Here's how the part is built. I have some questions about the finished solid (model axes, mm). A direction names the side the tool comes from. Give positions to 0.01 mm unless a question says otherwise; leave off trailing zeros. Loops run counter-clockwise (first coordinate to the right, second up) from the corner with the lowest first, then second, coordinate; pieces in that order, holes last.
Q1. If we section it at C-C (y = 32): Please give me the cut outline in (x, z) (3 decimals).
Q2. If we section it at D-D (z = -35.5): Please give me the cut outline in (x, y), plus the area to 3 significant figures.
Q3. If we section it at A-A (x = -12.5): Please give me the cut outline in (y, z) (3 decimals).
Q4. I need wall thicknesses on line 1 (X direction, y = 15, z = -4); line 2 (X direction, y = 8, z = -10); line 3 (Y direction, x = -12.5, z = -7.9). Which ranges of each line are inside material? Lowest first, please.
Q5. For faces 1 (the face through (-5, 13, -7.1)), 2 (the face through (-48, 28, -162)), 3 (the face through (-47, 28, -3)), 4 (the face through (-30, 32, -8)), which set-ups out of +Z, -Z, +X, -X, +Y, -Y let a thin tool reach every point of the face, with its end or its side?
Q6. We'd pull the mould along Y, two halves only. Please class faces 5 (the face through (-50, 33.75, -8)), 6 (the face through (-2, 13, -84)), 7 (the face through (-30, 32, -157)), 8 (the face through (-35, 30, -165)): +Y half, -Y half, draft (parallel to the pull), parting line (faces both ways), or undercut.
Q7. If we section it at B-B (y = 15.5): Give the number of separate pieces and of enclosed holes in the cut face, plus the area to 3 significant figures.
Q8. Will these pins go through, and if not, where does the flat tip stop? P1, Ø1, axis at x = -18.5, y = 7.5, coming from the -Z side; P2, Ø2.5, axis at x = -1, z = -106, coming from the +Y side; P3, Ø12, axis at y = 15, z = -90.5, coming from the -X side.
Autodesk Inventor part; units mm, degrees
ref_plane "YZ Plane" through (0, 0, 0) normal (1, 0, 0) x (0, 1, 0)
ref_plane "XZ Plane" through (0, 0, 0) normal (0, 1, 0) x (-1, 0, 0)
ref_plane "XY Plane" through (0, 0, 0) normal (0, 0, 1) x (1, 0, 0)
sketch "Sketch1" plane through (0, 0, 0) normal (0, 1, 0) x (-1, 0, 0)
  line L0 (0, 0) -> (25, 0)
  line L1 (25, 0) -> (25, -165)
  line L2 (25, -165) -> (0, -165)
  line L3 (0, -165) -> (0, 0)
  dimension "d0" = 25
  dimension "d1" = 165
extrude "Extrusion1" add sketch "Sketch1" along normal blind 3
sketch "Sketch2" plane through (0, 3, 0) normal (0, 1, 0) x (1, 0, 0)
  line L0 (0, 0) -> (0, 165)
  line L1 (-25, 165) -> (-25, 0)
  line L2 (0, 0) -> (-25, 0)
  line L3 (-25, 0) -> (-25, 8.5)
  line L4 (-25, 8.5) -> (0, 8.5)
  line L5 (0, 8.5) -> (0, 0)
  line L6 (-25, 165) -> (0, 165)
  line L7 (0, 165) -> (0, 156.5)
  line L8 (0, 156.5) -> (-25, 156.5)
  line L9 (-25, 156.5) -> (-25, 165)
  dimension "d4" = 8.5
  dimension "d5" = 8.5
extrude "Extrusion2" add sketch "Sketch2" along normal blind 25 contours L2 L1 L4 L0 | L8 L1 L6 L0
sketch "Sketch3" plane through (-25, 0, 0) normal (0, 0, 1) x (1, 0, 0)
  line L0 (0, 3) -> (0, 28) construction
  line L1 (25, 3) -> (25, 28) construction
  line L2 (0, 28) -> (25, 28) construction
  line L3 (25, 28) -> (25, 3) construction
  line L4 (25, 3) -> (0, 3) construction
  line L5 (0, 3) -> (0, 28) construction
  circle A0 centre (12.5, 15.5) radius 11
  point P0 (25, 0)
  dimension "d8" = 25
  dimension "d9" = 22
extrude "Extrusion3" cut sketch "Sketch3" against normal blind 7.1
sketch "Sketch4" plane through (-25, 0, 0) normal (0, 0, 1) x (1, 0, 0)
  circle A0 centre (12.5, 15.5) radius 11
  circle A1 centre (12.5, 15.5) radius 7.75
  point P0 (25, 0)
  dimension "d12" = 15.5
extrude "Extrusion4" cut sketch "Sketch4" against normal blind 165 contours A1
sketch "Sketch5" plane through (0, 0, -165) normal (0, 0, -1) x (-1, 0, 0)
  circle A0 centre (12.5, 15.5) radius 7.75
  circle A1 centre (12.5, 15.5) radius 11
  point P0 (0, 0)
extrude "Extrusion5" cut sketch "Sketch5" against normal blind 7.1
sketch "Sketch6" plane through (0, 3, 0) normal (0, 1, 0) x (1, 0, 0)
  line L0 (-25, 156.5) -> (-25, 8.5)
  line L1 (-20.25, 8.5) -> (-4.75, 8.5)
  line L2 (-25, 156.5) -> (-20, 156.5)
  line L3 (-20, 156.5) -> (-20, 8.5)
  line L4 (-20, 8.5) -> (-25, 8.5)
  line L5 (-25, 8.5) -> (-25, 156.5)
  line L6 (0, 8.5) -> (0, 156.5)
  line L7 (-4.75, 156.5) -> (-20.25, 156.5)
  line L8 (0, 8.5) -> (-5, 8.5)
  line L9 (-5, 8.5) -> (-5, 156.5)
  line L10 (-5, 156.5) -> (0, 156.5)
  line L11 (0, 156.5) -> (0, 8.5)
  point P0 (0, 0)
  dimension "d17" = 5
  dimension "d18" = 5
extrude "Extrusion6" add sketch "Sketch6" along normal blind 10 contours L2 L3 L1 L4 L0 | L7 L10 L6 L8 L1 L9
fillet "Fillet1" radius 2 2 edges at (-5, 13, -82.5) (-20, 13, -82.5)
sketch "Sketch7" plane through (-25, 0, 0) normal (0, 0, 1) x (1, 0, 0)
  point P0 (25, 0)
sketch "Sketch8" plane through (-25, 0, 0) normal (0, 0, 1) x (1, 0, 0)
  circle A0 centre (12.5, 15.5) radius 11
  circle A1 centre (12.5, 15.5) radius 11
  circle A2 centre (12.5, 15.5) radius 11.375
  point P0 (25, 0)
  dimension "d22" = 22.75
extrude "Extrusion7" cut sketch "Sketch8" against normal blind 7.1
sketch "Sketch9" plane through (0, 0, -165) normal (0, 0, -1) x (-1, 0, 0)
  circle A0 centre (12.5, 15.5) radius 11.375
  circle A1 centre (12.5, 15.5) radius 11.375
  point P0 (0, 0)
extrude "Extrusion8" cut sketch "Sketch9" against normal blind 7.1
sketch "Sketch10" plane through (-25, 0, -165) normal (-1, 0, 0) x (0, 0, 1)
  point P0 (165, 0)
sketch "Sketch11" plane through (-25, 0, -165) normal (-1, 0, 0) x (0, 0, 1)
  line L0 (165, 0) -> (0, 0)
  line L1 (0, 0) -> (16, 0)
  line L2 (16, 0) -> (16, 8)
  line L3 (16, 8) -> (0, 8)
  line L4 (0, 8) -> (0, 0)
  line L5 (165, 0) -> (149, 0)
  line L6 (149, 0) -> (149, 8)
  line L7 (149, 8) -> (165, 8)
  line L8 (165, 8) -> (165, 0)
  line L9 (8.5, 28) -> (0, 28)
  line L10 (0, 28) -> (16, 28)
  line L11 (16, 28) -> (16, 36)
  line L12 (16, 36) -> (0, 36)
  line L13 (0, 36) -> (0, 28)
  line L14 (165, 28) -> (156.5, 28)
  line L15 (165, 28) -> (149, 28)
  line L16 (149, 28) -> (149, 36)
  line L17 (149, 36) -> (165, 36)
  line L18 (165, 36) -> (165, 28)
  dimension "d27" = 16
  dimension "d28" = 8
  dimension "d29" = 16
  dimension "d30" = 16
  dimension "d31" = 8
  dimension "d32" = 16
extrude "Extrusion9" add sketch "Sketch11" along normal blind 45
sketch "Sketch12" plane through (0, 28, 0) normal (0, 1, 0) x (1, 0, 0)
  line L0 (-25, 0) -> (-70, 0)
  line L1 (0, 0) -> (-70, 0)
  line L2 (-25, 0) -> (0, 0)
  line L3 (0, 0) -> (0, 8.5)
  line L4 (0, 0) -> (0, 8.5)
  line L5 (-25, 16) -> (-25, 0)
  line L6 (0, 8.5) -> (-25, 16)
  line L7 (-25, 16) -> (-25, 0)
  line L8 (-25, 16) -> (-25, 149)
  line L9 (0, 156.5) -> (0, 165)
  line L10 (-25, 149) -> (0, 156.5)
  line L11 (0, 156.5) -> (0, 165)
  line L12 (-70, 165) -> (0, 165)
  line L13 (0, 165) -> (-25, 165)
  line L14 (-25, 149) -> (-25, 165)
extrude "Extrusion10" add sketch "Sketch12" along normal blind 8
sketch "Sketch13" plane through (-70, 0, -165) normal (-1, 0, 0) x (0, 0, 1)
  line L0 (0, 8) -> (16, 8) construction
  line L1 (0, 0) -> (16, 0) construction
  line L2 (0, 8) -> (16, 0) construction
  line L3 (14.125, 2.25) -> (1.875, 2.25)
  line L4 (1.875, 2.25) -> (1.875, 5.75)
  line L5 (1.875, 5.75) -> (14.125, 5.75)
  line L6 (14.125, 5.75) -> (14.125, 2.25)
  line L7 (14.125, 2.25) -> (1.875, 5.75) construction
  line L8 (1.875, 2.25) -> (14.125, 5.75) construction
  line L9 (0, 0) -> (0, 36) construction
  line L10 (16, 28) -> (8.5, 28) construction
  line L11 (0, 36) -> (16, 28) construction
  line L12 (14.125, 30.25) -> (1.875, 30.25)
  line L13 (1.875, 30.25) -> (1.875, 33.75)
  line L14 (1.875, 33.75) -> (14.125, 33.75)
  line L15 (14.125, 33.75) -> (14.125, 30.25)
  line L16 (14.125, 30.25) -> (1.875, 33.75) construction
  line L17 (1.875, 30.25) -> (14.125, 33.75) construction
  line L18 (149, 0) -> (149, 8) construction
  line L19 (0, 0) -> (165, 0) construction
  line L20 (149, 8) -> (165, 0) construction
  line L21 (165, 36) -> (149, 36) construction
  line L22 (149, 28) -> (165, 28) construction
  line L23 (149, 36) -> (165, 28) construction
  line L24 (163.125, 30.25) -> (150.875, 30.25)
  line L25 (150.875, 30.25) -> (150.875, 33.75)
  line L26 (150.875, 33.75) -> (163.125, 33.75)
  line L27 (163.125, 33.75) -> (163.125, 30.25)
  line L28 (163.125, 30.25) -> (150.875, 33.75) construction
  line L29 (150.875, 30.25) -> (163.125, 33.75) construction
  line L30 (163.125, 2.25) -> (150.875, 2.25)
  line L31 (150.875, 2.25) -> (150.875, 5.75)
  line L32 (150.875, 5.75) -> (163.125, 5.75)
  line L33 (163.125, 5.75) -> (163.125, 2.25)
  line L34 (163.125, 2.25) -> (150.875, 5.75) construction
  line L35 (150.875, 2.25) -> (163.125, 5.75) construction
  point P0 (8, 4)
  point P1 (8, 32)
  point P2 (157, 32)
  point P3 (157, 4)
  dimension "d37" = 12.25
  dimension "d38" = 3.5
  dimension "d39" = 12.25
  dimension "d40" = 3.5
  dimension "d41" = 12.25
  dimension "d42" = 3.5
  dimension "d43" = 12.25
extrude "Extrusion11" cut sketch "Sketch13" against normal blind 40
sketch "Sketch14" plane through (-25, 8, -149) normal (0, 1, 0) x (1, 0, 0)
  line L0 (0, 16) -> (0, 0) construction
  line L1 (0, 8) -> (0, 10.5) construction
  line L2 (-45, 0) -> (-45, 16)
  line L3 (0, 10.5) -> (-45, 10.5)
  line L4 (-45, 10.5) -> (-45, 5.5)
  line L5 (-45, 5.5) -> (0, 5.5)
  line L6 (0, 5.5) -> (0, 10.5)
  line L7 (0, -133) -> (0, -149) construction
  line L8 (0, -141) -> (0, -143.5) construction
  line L9 (-45, -149) -> (-45, -133)
  line L10 (0, -143.5) -> (-45, -143.5)
  line L11 (-45, -143.5) -> (-45, -138.5)
  line L12 (-45, -138.5) -> (0, -138.5)
  line L13 (0, -138.5) -> (0, -143.5)
  point P0 (25, -149)
  dimension "d46" = 2.5
  dimension "d47" = 5
  dimension "d48" = 2.5
  dimension "d49" = 5
extrude "Extrusion12" add sketch "Sketch14" along normal blind 20
properties part number "frontAxelHolder 10-23"
Check sheet entries:
1. outline: (-70, -165) - (0, -165) - (0, -156.5) - (-25, -149) - (-70, -149) - (-70, -150.875) - (-30, -150.875) - (-30, -163.125) - (-70, -163.125) - close; (-70, -16) - (-25, -16) - (0, -8.5) - (0, 0) - (-70, 0) - (-70, -1.875) - (-30, -1.875) - (-30, -14.125) - (-70, -14.125) - close
2. outline: (-25, 0) - (0, 0) - (0, 13) - (-3, 13) arc R2 ccw to (-5, 11) - (-5, 3) - (-20, 3) - (-20, 11) arc R2 ccw to (-22, 13) - (-25, 13) - close
2. area: 173 mm2
3. outline: (0, -165) - (4.125, -165) - (4.125, -157.9) - (7.75, -157.9) - (7.75, -156.5) - (3, -156.5) - (3, -8.5) - (7.75, -8.5) - (7.75, -7.1) - (4.125, -7.1) - (4.125, 0) - (0, 0) - close; (23.25, -157.9) - (26.875, -157.9) - (26.875, -165) - (36, -165) - (36, -152.75) - (28, -152.75) - (28, -156.5) - (23.25, -156.5) - close; (23.25, -8.5) - (28, -8.5) - (28, -12.25) - (36, -12.25) - (36, 0) - (26.875, 0) - (26.875, -7.1) - (23.25, -7.1) - close
4. line 1: x = -25 to -23.86, -1.14 to 0
4. line 2: x = -70 to -20, -5 to 0
4. line 3: y = 0 to 7.75, 23.25 to 36
5. face 1: +Z
5. face 2: -Z, -X
5. face 3: +Z, -X
5. face 4: -X
6. face 5: undercut
6. face 6: +Y half
6. face 7: undercut
6. face 8: draft
7. separate pieces: 4
7. enclosed holes: 0
7. area: 509 mm2
8. P1: stops at z = -157.9
8. P2: stops at y = 13
8. P3: stops at x = -25
